Autodesk Fusion 360 part; units mm, degrees
sketch "Sketch1" plane through (0, 0, 0) normal (0, 0, 1) x (1, 0, 0)
  line L0 (2, 0) -> (128, 0)
  line L1 (130, 2) -> (130, 18)
  line L2 (128, 20) -> (2, 20)
  line L3 (0, 18) -> (0, 2)
  arc A0 (2, 20) -> (0, 18) centre (2, 18) ccw
  arc A1 (0, 2) -> (2, 0) centre (2, 2) ccw
  arc A2 (128, 0) -> (130, 2) centre (128, 2) ccw
  arc A3 (130, 18) -> (128, 20) centre (128, 18) ccw
  line L4 (4, 4) -> (126, 4)
  line L5 (126, 4) -> (126, 16)
  line L6 (126, 16) -> (4, 16)
  line L7 (4, 16) -> (4, 4)
  line L8 (22.5, 16) -> (27.5, 16)
  line L9 (27.5, 16) -> (27.5, 4)
  line L10 (27.5, 4) -> (22.5, 4)
  line L11 (22.5, 4) -> (22.5, 16)
  line L12 (65, 0) -> (65, 20) construction
  line L13 (107.5, 4) -> (107.5, 16)
  line L14 (107.5, 16) -> (102.5, 16)
  line L15 (102.5, 4) -> (107.5, 4)
  line L16 (102.5, 16) -> (102.5, 4)
  line L17 (22.5, 12.75) -> (107.5, 12.75)
  line L18 (107.5, 12.75) -> (107.5, 7.25)
  line L19 (107.5, 7.25) -> (22.5, 7.25)
  line L20 (22.5, 7.25) -> (22.5, 12.75)
  line L21 (22.5, 12.75) -> (107.5, 7.25) construction
  line L22 (107.5, 12.75) -> (22.5, 7.25) construction
  line L23 (9, 4) -> (9, 16)
  line L24 (121, 4) -> (121, 16)
  point P0 (130, 0)
  point P1 (0, 20)
  point P2 (65, 10)
  dimension "d1" = 130
  dimension "d2" = 20
  dimension "d3" = 2
  dimension "d4" = -4
  dimension "d5" = 5
  dimension "d7" = 80
  dimension "d16" = 5.5
  dimension "d23" = 5
  dimension "d24" = 5
extrude "Extrude1" add sketch "Sketch1" along normal blind 4 contours L0 L1 L2 L3 A0 A1 A2 A3 | L4 L9 L10 L11 L19 | L9 L11 L17 L19 L20 | L6 L8 L9 L11 L17 | L4 L13 L15 L16 L19 | L13 L16 L17 L18 L19 | L6 L13 L14 L16 L17
extrude "Extrude3" add sketch "Sketch1" against normal blind 4 contours L9 L11 L17 L19 L20 | L13 L16 L17 L18 L19
fillet "Fillet1" radius 1 4 edges at (25, 12.75, -4) (25, 7.25, -4) (105, 12.75, -4) (105, 7.25, -4)
fillet "Fillet2" radius 2 12 edges at (126, 4, 2) (107.5, 4, 2) (102.5, 4, 2) (126, 16, 2) (107.5, 16, 2) (102.5, 16, 2) (22.5, 4, 2) (4, 4, 2) (4, 16, 2) (22.5, 16, 2) (27.5, 4, 2) (27.5, 16, 2)
extrude "Extrude4" add sketch "Sketch1" against normal blind 0.2 from surface at 4 contours L4 L6 L7 L23 | L4 L5 L6 L24
Geometry check sheet. Reference: the model listing, model coordinates, mm. A direction names the side the tool comes from. Round coordinates to 2 decimals unless told otherwise and drop trailing zeros. Write each loop counter-clockwise with the first axis right and the second up, starting at its lowest first coordinate (ties: lowest second). Pieces come first, ordered by that corner, then holes. Notation, with made-up numbers: (18.5, 59) - (71.5, 59) arc R30 ccw to (71.5, 94) - close; hole circle Ø7 at (9, 6.25). An arc over 180 degrees is marked (long way). Write each question's results on one line, items separated by ' | '.
(1) Depth check by flat-ended pin: pin 1 Ø5.5 at (x, y) = (6.5, 9.5) entering from -Z; pin 2 Ø2.5 at (x, z) = (25.5, -2) entering from -Y; pin 3 Ø3 at (y, z) = (9, 1) entering from -X; pin 4 Ø4 at (x, y) = (77, 6.5) entering from +Z. Enter the tip coordinate at first touch or a pass-through.
Computed:
pin 1: stops at z = 0 | pin 2: stops at y = 7.25 | pin 3: stops at x = 0 | pin 4: passes through
(2) Set-up check for faces 5 (the face through (6, 10, 3.8)), 6 (the face through (65, 4, 2)), 7 (the face through (105, 10, -4)): record each of +Z, -Z, +X, -X, +Y, -Y from which the full face is reachable in a straight line by a thin tool's end or side.
Computed:
face 5: -Z | face 6: +Z, -Z | face 7: -Z, +X, -X, +Y, -Y
(3) Sectioned sample at B-B, the plane z = 1.25. Count the separate pieces of the cut face and the enclosed holes in it, plus the area to 3 significant figures.
Computed:
separate pieces: 1 | enclosed holes: 3 | area: 1,260 mm^2
(4) Draft check along Y on faces 1 (the face through (125.43, 15.4, 1.93)), 2 (the face through (0.57, 19.4, 1.97)), 3 (the face through (130, 10, 2)), 4 (the face through (25, 7.25, -1)). Enter one of: pulls with the +Y half, pulls with the -Y half, needs draft (parallel to the pull), parting line crosses it, or undercut.
Computed:
face 1: undercut | face 2: pulls with the +Y half | face 3: needs draft | face 4: pulls with the -Y half
(5) Thickness scan on probe 1 along X at (y, z) = (11.25, 1.5); probe 2 along Y at (x, z) = (36, 1.5); probe 3 along X at (y, z) = (5, 3). Record the ranges inside material, lowest first. Write a range as from..to.
Computed:
probe 1: x = 0..4, 22.5..27.5, 102.5..107.5, 126..130 | probe 2: y = 0..4, 16..20 | probe 3: x = 0..4.27, 22.23..27.77, 102.23..107.77, 125.73..130
(6) Sectioned sample at A-A, the plane x = 58. Enter the section's corners in (y, z).
Computed:
outline: (0, 0) - (4, 0) - (4, 4) - (0, 4) - close; (16, 0) - (20, 0) - (20, 4) - (16, 4) - close
